For this review, take the finished solid that the model builds, in its own axes (mm). A direction names the side the tool comes from. Give positions to 0.01 mm unless a question says otherwise; leave off trailing zeros. Order: outer loops, then holes, each group sorted by start corner. A loop starts at its lowest first (then second) coordinate and runs counter-clockwise, first axis right, second up. Notation, with made-up numbers: M 9.5,-9 L 44.5,-9 A22 ccw 44.5,9 Z; hole C 23.5,21.25 d3. An arc over 180 degrees is marked long. Answer as CSV lines item,"result". Start each with the question number.
1. We need section A-A, the plane y = 6. Give the boundary of the cut face in (x, z), and give its area (3 significant figures).
2. We need section C-C, the plane z = 6.25. Give the boundary of the cut face in (x, y), and give its area (3 significant figures).
3. Machinability: for faces 1 (the cylindrical face through (-0.3, 6.3, 5.8)), 2 (the flat face through (1.8, -3.42, 3.87)), 3 (the flat face through (0, 6, -4.039)), which of the approach directions +Z, -Z, +X, -X, +Y, -Y give a long, thin tool a straight path to every point of the face, cutting with its end or side? Answer none if there is none.
4. We need section B-B, the plane z = 1.5. Give the boundary of the cut face in (x, y).
5. Clearance check with flat-ended pins moving along their axes: P1, Ø2.5, axis at x = 1, z = -1, coming from the +Y side; P2, Ø3, axis at x = 0, y = -4.445, coming from the -Z side; P3, Ø4, axis at x = 3.5, y = 0, coming from the -Z side; P4, Ø2.5, axis at x = -1, y = 4.5, coming from the +Z side. State where each tip first meets the part, or that it passes through.
6. We need section D-D, the plane x = 0. State how many separate pieces and enclosed holes the cut face has, and give its area (3 significant figures).
7. Mouldability with a two-part tool opening along X and no side actions: class faces 4 (the flat face through (2, 0, 5)), 5 (the flat face through (0, 6, 4.039)), 6 (the cylindrical face through (-2.731, -4.383, -4.283)) as pulls with the +X half, pulls with the -X half, needs draft (parallel to the pull), parting line crosses it, or undercut.
8. For line 1 along Y through (x, z) = (0, 5.6); line 2 along Y through (x, z) = (-0.25, -5); line 3 along X through (y, z) = (-4.5, 0), list the stretches that pass through material, from the lowest coordinate up.
from build123d import *

# Parameters (mm, degrees)
SKETCH1_R               = 7.62
BOSS_EXTRUDE1_DEPTH     = 10
CUT_EXTRUDE1_DEPTH      = 7.62
SKETCH4_R               = 2.75
CUT_EXTRUDE2_DEPTH      = 9.5
SKETCH5_R               = 5.08
BOSS_EXTRUDE2_DEPTH     = 8.89
CUT_EXTRUDE3_REACH      = 20.89
SKETCH6_R               = 2.08915
SKETCH7_R               = 1.1
CUT_EXTRUDE4_DEPTH      = 8.89
CUT_EXTRUDE4_DEPTH_BACK = 8.89
SKETCH8_R               = 1.2
CUT_EXTRUDE5_DEPTH      = 8.89
CUT_EXTRUDE5_DEPTH_BACK = 8.89
CUT_EXTRUDE6_DEPTH      = 1.905


with BuildPart() as part:
    # Sketch1 → Boss-Extrude1 (new body)
    with BuildSketch(Plane(origin=(0, 0, 0), x_dir=(1, 0, 0), z_dir=(0, 1, 0))):
        Circle(SKETCH1_R)
    extrude(amount=BOSS_EXTRUDE1_DEPTH)

    # Sketch2 → Cut-Extrude1 (cut)
    with BuildSketch(Plane(origin=(0, 10, 0), x_dir=(1, 0, 0), z_dir=(0, 1, 0))):
        Polygon((-2.331686797, 4.0386), (-4.663373594, 0), (-2.331686797, -4.0386), (2.331686797, -4.0386), (4.663373594, 0), (2.331686797, 4.0386), align=None)
    extrude(amount=-CUT_EXTRUDE1_DEPTH, mode=Mode.SUBTRACT)

    # Sketch4 → Cut-Extrude2 (cut)
    with BuildSketch(Plane(origin=(0, 2.38, 0), x_dir=(1, 0, 0), z_dir=(0, 1, 0))):
        Circle(SKETCH4_R)
    extrude(amount=-CUT_EXTRUDE2_DEPTH, mode=Mode.SUBTRACT)

    # Sketch5 → Boss-Extrude2 (add)
    with BuildSketch(Plane(origin=(0, 0, 0), x_dir=(-1, 0, 0), z_dir=(0, -1, 0))):
        Circle(SKETCH5_R)
    extrude(amount=BOSS_EXTRUDE2_DEPTH)

    # Sketch6 → Cut-Extrude3 (cut, up to next)
    with BuildSketch(Plane(origin=(0, -8.89, 0), x_dir=(-1, 0, 0), z_dir=(0, -1, 0)), mode=Mode.PRIVATE) as cut_extrude3_sk1:
        Circle(SKETCH6_R)
    cut_extrude3_tool1 = extrude(cut_extrude3_sk1.sketch, amount=-CUT_EXTRUDE3_REACH, mode=Mode.PRIVATE) & part.part
    add(cut_extrude3_tool1.solids().sort_by_distance((0, -8.89, 0))[0], mode=Mode.SUBTRACT)

    # Sketch7 → Cut-Extrude4 (cut, two sides)
    with BuildSketch(Plane.XY) as cut_extrude4_sk:
        with Locations((0, -4.445)):
            Circle(SKETCH7_R)
    extrude(amount=CUT_EXTRUDE4_DEPTH, mode=Mode.SUBTRACT)
    extrude(cut_extrude4_sk.sketch, amount=-CUT_EXTRUDE4_DEPTH_BACK, mode=Mode.SUBTRACT)

    # Sketch8 → Cut-Extrude5 (cut, two sides)
    with BuildSketch(Plane.XY) as cut_extrude5_sk:
        with Locations((0, 7.46)):
            Circle(SKETCH8_R)
    extrude(amount=CUT_EXTRUDE5_DEPTH, mode=Mode.SUBTRACT)
    extrude(cut_extrude5_sk.sketch, amount=-CUT_EXTRUDE5_DEPTH_BACK, mode=Mode.SUBTRACT)

    # Sketch9 → Cut-Extrude6 (cut)
    with BuildSketch(Plane.XY.offset(5.08)):
        Polygon((1.195172792, -2.3749), (-1.195172792, -2.3749), (-2.390345584, -4.445), (-1.195172792, -6.5151), (1.195172792, -6.5151), (2.390345584, -4.445), align=None)
    extrude(amount=-CUT_EXTRUDE6_DEPTH, mode=Mode.SUBTRACT)


solid = part.part
Result set:
1,outline,"C 0,0 d15.24; hole M -4.66,0 L -2.33,-4.04 L 2.33,-4.04 L 4.66,0 L 2.33,4.04 L -2.33,4.04 Z"
1,area,"126 mm2"
2,outline,"M -4.36,0 L 4.36,0 L 4.36,10 L -4.36,10 Z; hole C 0,7.46 d2.4"
2,area,"82.7 mm2"
3,face 1,"+Z, -Z"
3,face 2,"+Z"
3,face 3,"+Y"
4,outline,"M -7.47,0 L -4.85,0 L -4.85,-8.89 L -1.45,-8.89 L -1.45,0 L -2.3,0 L -2.3,2.38 L -3.8,2.38 L -3.8,10 L -7.47,10 Z; M 1.45,-8.89 L 4.85,-8.89 L 4.85,0 L 7.47,0 L 7.47,10 L 3.8,10 L 3.8,2.38 L 2.3,2.38 L 2.3,0 L 1.45,0 Z"
5,P1,"y = 0"
5,P2,"z = -5.08"
5,P3,"z = -7.47"
5,P4,"z = 7.62"
6,separate pieces,"6"
6,enclosed holes,"0"
6,area,"96.9 mm2"
7,face 4,"needs draft"
7,face 5,"undercut"
7,face 6,"parting line crosses it"
8,line 1,"0 to 6.26, 8.66 to 10"
8,line 2,"-8.89 to -5.52, -3.37 to 6.29, 8.63 to 10"
8,line 3,"-5.08 to -2.09, 2.09 to 5.08"
